```python
from build123d import *

# Parameters (mm, degrees)
F0_W     = 18.415
F0_H     = 3.81
F1_DEPTH = 17.78
F2_R     = 5.842
F2_R_2   = 3.2385
F3_DEPTH = 25.4
F4_R     = 5.842
F4_R_2   = 3.175
F5_DEPTH = 25.4
F6_DEPTH = 11.43
F7_DEPTH = 6.7437
F8_DEPTH = 11.43


with BuildPart() as f1:
    # F0 (on Top) → F1 (new body)
    with BuildSketch(Plane.XY):
        with BuildLine():
            ThreePointArc((-40.741389, 181.9), (-47.281889, 175.3595), (-53.822389, 181.9))
            Line((-53.822389, 181.9), (-53.822389, 184.44))
            ThreePointArc((-53.822389, 184.44), (-55.310286, 188.032102), (-58.902389, 189.52))
            Line((-58.902389, 189.52), (-60.172389, 189.52))
            ThreePointArc((-60.172389, 189.52), (-61.96844, 188.776051), (-62.712389, 186.98))
            Line((-62.712389, 186.98), (-62.712389, 174.28))
            Line((-62.712389, 174.28), (-11.405862, -20.666177))
            ThreePointArc((-11.405862, -20.666177), (-9.141817, -24.079176), (-5.264977, -25.4))
            Line((-5.264977, -25.4), (-2.54, -25.4))
            Line((-2.54, -25.4), (0, -25.4))
            Line((0, -25.4), (0, -3.175))
            ThreePointArc((0, -3.175), (-2.245064, 2.245064), (3.175, 0))
            Line((3.175, 0), (3.175, 3.81))
            Line((3.175, 3.81), (21.59, 3.81))
            ThreePointArc((21.59, 3.81), (22.333949, 5.606051), (24.13, 6.35))
            Line((24.13, 6.35), (33.528, 6.35))
            ThreePointArc((33.528, 6.35), (35.324051, 5.606051), (36.068, 3.81))
            Line((36.068, 3.81), (52.249596, 3.81))
            Line((52.249596, 3.81), (-31.175642, 188.02783))
            ThreePointArc((-31.175642, 188.02783), (-32.112828, 189.114606), (-33.489438, 189.52))
            Line((-33.489438, 189.52), (-35.661389, 189.52))
            ThreePointArc((-35.661389, 189.52), (-39.253491, 188.032102), (-40.741389, 184.44))
            Line((-40.741389, 184.44), (-40.741389, 181.9))
        make_face()
        with BuildLine():
            Line((12.199936, 59.813391), (-7.329708, 21.209695))
            ThreePointArc((-7.329708, 21.209695), (-9.863664, 19.830428), (-12.052532, 21.709833))
            Line((-12.052532, 21.709833), (-22.21237, 60.313529))
            ThreePointArc((-22.21237, 60.313529), (-21.767686, 62.510736), (-19.756016, 63.5))
            Line((-19.756016, 63.5), (9.933466, 63.5))
            ThreePointArc((9.933466, 63.5), (12.097258, 62.290265), (12.199936, 59.813391))
        make_face(mode=Mode.SUBTRACT)
        with BuildLine():
            Line((26.073642, 15.24), (5.167911, 15.24))
            ThreePointArc((5.167911, 15.24), (3.004119, 16.449735), (2.901441, 18.926609))
            Line((2.901441, 18.926609), (17.049915, 46.893498))
            ThreePointArc((17.049915, 46.893498), (19.37115, 48.286298), (21.630181, 46.794719))
            Line((21.630181, 46.794719), (31.858132, 24.209575))
            ThreePointArc((31.858132, 24.209575), (31.410158, 18.148474), (26.073642, 15.24))
        make_face(mode=Mode.SUBTRACT)
        with BuildLine():
            Line((-9.022239, 106.675746), (-22.704861, 79.629695))
            ThreePointArc((-22.704861, 79.629695), (-25.238817, 78.250428), (-27.427685, 80.129833))
            Line((-27.427685, 80.129833), (-34.545747, 107.175885))
            ThreePointArc((-34.545747, 107.175885), (-34.101063, 109.373091), (-32.089393, 110.362355))
            Line((-32.089393, 110.362355), (-11.288709, 110.362355))
            ThreePointArc((-11.288709, 110.362355), (-9.124918, 109.152621), (-9.022239, 106.675746))
        make_face(mode=Mode.SUBTRACT)
        with BuildLine():
            ThreePointArc((-13.383049, 124.110186), (-13.562239, 121.685745), (-15.696845, 120.522355))
            Line((-15.696845, 120.522355), (-24.116154, 120.522355))
            ThreePointArc((-24.116154, 120.522355), (-26.279946, 121.73209), (-26.382624, 124.208965))
            Line((-26.382624, 124.208965), (-21.940091, 132.990396))
            ThreePointArc((-21.940091, 132.990396), (-19.618855, 134.383196), (-17.359824, 132.891616))
            Line((-17.359824, 132.891616), (-13.383049, 124.110186))
        make_face(mode=Mode.SUBTRACT)
        with BuildLine():
            Line((-39.761062, 126.992189), (-47.664299, 157.021619))
            ThreePointArc((-47.664299, 157.021619), (-47.283962, 159.131562), (-45.424544, 160.198838))
            ThreePointArc((-45.424544, 160.198838), (-39.847134, 161.427711), (-34.780915, 164.064198))
            ThreePointArc((-34.780915, 164.064198), (-32.65263, 164.43414), (-31.009279, 163.032051))
            Line((-31.009279, 163.032051), (-24.933857, 149.616433))
            ThreePointArc((-24.933857, 149.616433), (-24.595436, 147.962539), (-25.004845, 146.324773))
            Line((-25.004845, 146.324773), (-35.038238, 126.49205))
            ThreePointArc((-35.038238, 126.49205), (-37.572194, 125.112783), (-39.761062, 126.992189))
        make_face(mode=Mode.SUBTRACT)
        with BuildLine():
            Line((5.525331, 73.66), (-11.782777, 73.66))
            ThreePointArc((-11.782777, 73.66), (-13.946569, 74.869735), (-14.049247, 77.346609))
            Line((-14.049247, 77.346609), (-4.916449, 95.399154))
            ThreePointArc((-4.916449, 95.399154), (-2.595213, 96.791954), (-0.336183, 95.300374))
            Line((-0.336183, 95.300374), (7.839127, 77.24783))
            ThreePointArc((7.839127, 77.24783), (7.659937, 74.82339), (5.525331, 73.66))
        make_face(mode=Mode.SUBTRACT)
        Polygon((53.975, 0), (52.249596, 3.81), (36.068, 3.81), (36.068, 0), align=None)
        with Locations((12.3825, 1.905)):
            Rectangle(F0_W, F0_H)
    extrude(amount=-F1_DEPTH)

    # F2 (on face) → F3 (cut)
    with BuildSketch(Plane.YZ):
        with Locations((-14.2875, -8.89)):
            Circle(F2_R)
        with Locations((-14.2875, -8.89)):
            Circle(F2_R_2, mode=Mode.SUBTRACT)
        with Locations((-14.2875, -8.89)):
            Circle(F2_R_2)
    extrude(amount=-F3_DEPTH, mode=Mode.SUBTRACT)

    # F4 (on face) → F5 (cut)
    with BuildSketch(Plane.XZ):
        with Locations((12.7, -8.89)):
            Circle(F4_R)
        with Locations((12.7, -8.89)):
            Circle(F4_R_2, mode=Mode.SUBTRACT)
        with Locations((45.0215, -8.89)):
            Circle(F4_R)
        with Locations((45.0215, -8.89)):
            Circle(F4_R_2, mode=Mode.SUBTRACT)
        with Locations((12.7, -8.89)):
            Circle(F4_R_2)
        with Locations((45.0215, -8.89)):
            Circle(F4_R_2)
    extrude(amount=-F5_DEPTH, mode=Mode.SUBTRACT)

    # F4 (on face) → F6 (join)
    with BuildSketch(Plane.XZ):
        with Locations((12.7, -8.89)):
            Circle(F4_R)
        with Locations((12.7, -8.89)):
            Circle(F4_R_2, mode=Mode.SUBTRACT)
    extrude(amount=-F6_DEPTH)

    # F4 (on face) → F7 (join)
    with BuildSketch(Plane.XZ):
        with Locations((45.0215, -8.89)):
            Circle(F4_R)
        with Locations((45.0215, -8.89)):
            Circle(F4_R_2, mode=Mode.SUBTRACT)
    extrude(amount=-F7_DEPTH)

    # F2 (on face) → F8 (join)
    with BuildSketch(Plane.YZ):
        with Locations((-14.2875, -8.89)):
            Circle(F2_R)
        with Locations((-14.2875, -8.89)):
            Circle(F2_R_2, mode=Mode.SUBTRACT)
    extrude(amount=-F8_DEPTH)


solid = f1.part
```
Can you work these out from the model? Positions are in its coordinate system, mm. A direction names the side the tool comes from. Coordinates: 2 decimals unless noted, no trailing zeros. Order: outer loops, then holes, each group sorted by start corner. A loop starts at its lowest first (then second) coordinate and runs counter-clockwise, first axis right, second up. Notation, with made-up numbers: (89.5, -11.5) -> (128.5, -11.5) arc R24 cw to (128.5, 21.5) -> close; hole circle Ø9 at (62, -26). An arc over 180 degrees is marked (long way). Write each question's results on one line, items separated by ' | '.
Item 1: I'm going to push flat-ended pins straight in: pin 1 Ø1.9 at (y, z) = (2.5, -10.5) entering from +X; pin 2 Ø6 at (y, z) = (-14, -11) entering from -X; pin 3 Ø1.5 at (x, z) = (-5, -16) entering from +Y. Where does each tip first touch, or does it pass through?
Results are:
pin 1: x = 53.27 | pin 2: x = -11.43 | pin 3: y = 131.88
Item 2: I want a section at C-C, the plane z = -8.89. Count the separate pieces of the cut face and the enclosed holes in it, then the cut area to 3 significant figures.
Results are:
separate pieces: 3 | enclosed holes: 5 | area: 6,650 mm²
Item 3: If we mould it in two halves opening along Y, with no side actions, what happens to faces 1 (the face through (-3, 73.66, -9)), 2 (the face through (-55.27, 187.99, -8.77)), 3 (the face through (10.18, 5.63, -10.82)), 4 (the face through (-3, -25.4, -9))? For each: +Y half, -Y half, draft (parallel to the pull), parting line (faces both ways), or undercut.
Results are:
face 1: undercut | face 2: +Y half | face 3: draft | face 4: -Y half
Item 4: I want a section at A-A, the plane y = 89.5. Write out the boundary of the cut face in (x, z), then the cut area to 3 significant figures.
Results are:
outline: (-40.4, -17.78) -> (-29.89, -17.78) -> (-29.89, 0) -> (-40.4, 0) -> close; (-17.71, -17.78) -> (-7.9, -17.78) -> (-7.9, 0) -> (-17.71, 0) -> close; (2.29, -17.78) -> (13.44, -17.78) -> (13.44, 0) -> (2.29, 0) -> close | area: 560 mm²
Item 5: I want a section at B-B, the plane y = 139. Write out the boundary of the cut face in (x, z).
Results are:
outline: (-53.43, -17.78) -> (-42.92, -17.78) -> (-42.92, 0) -> (-53.43, 0) -> close; (-28.71, -17.78) -> (-8.97, -17.78) -> (-8.97, 0) -> (-28.71, 0) -> close
Item 6: Which directions (+Z, -Z, +X, -X, +Y, -Y) give clear straight access to the entire face, cutting with the end or side of a thin tool? Please do faces 5 (the face through (-26.26, 121.7, -8.77)), 6 (the face through (-62.712, 181, -9)), 7 (the face through (-11.43, -11.8, -11.4)).
Results are:
face 5: +Z, -Z | face 6: +Z, -Z, -X, +Y, -Y | face 7: -X
Item 7: If I drill on line 1 along X through (y, z) = (96.5, -9.5); line 2 along Y through (x, z) = (6, -12.75); line 3 along X through (y, z) = (36, -16.75), over which ranges is the centre line in solid material (lowest first)?
Results are:
line 1: -42.24 to -31.74, -14.17 to -3.83, -1.47 to 10.27 | line 2: 0 to 15.24, 25.05 to 47.56, 63.5 to 73.7, 81.31 to 105.94 | line 3: -26.32 to -15.81, 0.15 to 11.54, 26.52 to 37.67
